Part model, mm, in its own coordinate system. Face numbers are marked on the shaded views. Coordinates: 2 decimals unless noted, no trailing zeros. Loops run counter-clockwise (first coordinate to the right, second up) from the corner with the lowest first, then second, coordinate; pieces in that order, holes last. Notation, with made-up numbers: (20.25, 4) -> (75.25, 4) arc R20 ccw to (75.25, 41) -> close; hole circle Ø10 at (23, -33.75). An arc over 180 degrees is marked (long way). One line per item, written item: value. Start each with the question number.
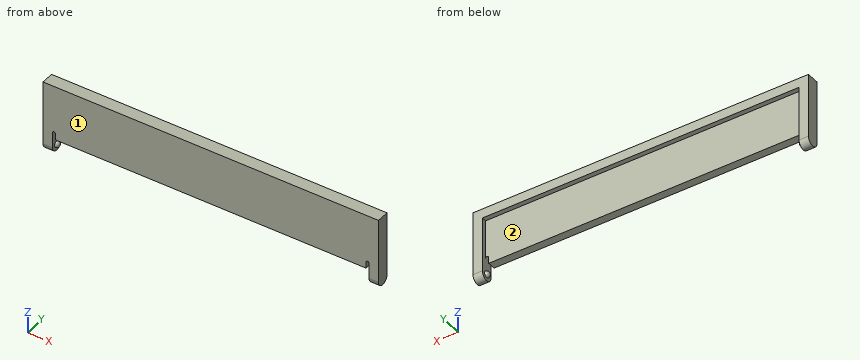
from build123d import *

# Parameters (mm, degrees)
SALIENTE_EXTRUIR1_DEPTH = 4
CROQUIS4_W              = 99
CROQUIS4_H              = 2
CORTAR_EXTRUIR1_DEPTH   = 10
REDONDEO1_R             = 2
CROQUIS5_W              = 101
CROQUIS5_H              = 16.071267716
CORTAR_EXTRUIR2_DEPTH   = 1.5


with BuildPart() as part:
    # Croquis1 → Saliente-Extruir1 (new body)
    with BuildSketch(Plane(origin=(0, 0, 0), x_dir=(1, 0, 0), z_dir=(0, 1, 0))):
        Polygon((-64.683943666, 30.054443615), (36.316056334, 30.054443615), (36.316056334, 33.054443615), (39.316056334, 33.054443615), (39.316056334, 30.054443615), (39.316056334, 10.554443615), (-67.683943666, 10.554443615), (-67.683943666, 30.054443615), (-67.683943666, 33.054443615), (-64.683943666, 33.054443615), align=None)
    extrude(amount=SALIENTE_EXTRUIR1_DEPTH)

    # Croquis4 → Cortar-Extruir1 (cut)
    with BuildSketch(Plane(origin=(0, 4, 0), x_dir=(1, 0, 0), z_dir=(0, 1, 0))):
        with Locations((-14.183943666, 29.054443615)):
            Rectangle(CROQUIS4_W, CROQUIS4_H)
        with BuildLine():
            Line((36.316056334, 26.054443615), (36.316056334, 30.054443615))
            Line((36.316056334, 30.054443615), (35.316056334, 30.054443615))
            Line((35.316056334, 30.054443615), (35.316056334, 28.054443615))
            Line((35.316056334, 28.054443615), (35.316056334, 26.054443615))
            ThreePointArc((35.316056334, 26.054443615), (35.816056334, 25.554443615), (36.316056334, 26.054443615))
        make_face()
        with BuildLine():
            Line((-63.683943666, 28.054443615), (-63.683943666, 30.054443615))
            Line((-63.683943666, 30.054443615), (-64.683943666, 30.054443615))
            Line((-64.683943666, 30.054443615), (-64.683943666, 26.054443615))
            ThreePointArc((-64.683943666, 26.054443615), (-64.183943666, 25.554443615), (-63.683943666, 26.054443615))
            Line((-63.683943666, 26.054443615), (-63.683943666, 28.054443615))
        make_face()
    extrude(amount=-CORTAR_EXTRUIR1_DEPTH, mode=Mode.SUBTRACT)

    # Redondeo1
    redondeo1_edges = [part.edges().sort_by_distance(p)[0] for p in [
        (-66.183943666, 0, -33.054443615),
        (-66.183943666, 4, -33.054443615),
        (37.816056334, 0, -33.054443615),
        (37.816056334, 4, -33.054443615),
    ]]
    fillet(redondeo1_edges, radius=REDONDEO1_R - 0.0001)  # a hair under: the kernel refuses the full size

    # Croquis3 → Revolución1 (revolve)
    with BuildSketch(Plane(origin=(-64.683943666, 0, 0), x_dir=(0, 0, -1), z_dir=(1, 0, 0))):
        with BuildLine():
            Line((32.054443615, 2), (30.054443615, 2))
            ThreePointArc((30.054443615, 2), (31.054443615, 1), (32.054443615, 2))
        make_face()
    revolve(axis=Axis((-64.683943666, 2, -32.054443615), (0, 0, 1)))

    # Croquis2 → Revolución2 (revolve)
    with BuildSketch(Plane.ZY.offset(-36.316056334)):
        with BuildLine():
            Line((-32.054443615, 2), (-30.054443615, 2))
            ThreePointArc((-30.054443615, 2), (-31.054443615, 1), (-32.054443615, 2))
        make_face()
    revolve(axis=Axis((36.316056334, 2, -32.054443615), (0, 0, 1)))

    # Croquis5 → Cortar-Extruir2 (cut)
    with BuildSketch(Plane(origin=(0, 4, 0), x_dir=(1, 0, 0), z_dir=(0, 1, 0))):
        with Locations((-14.183943666, 21.590077473)):
            Rectangle(CROQUIS5_W, CROQUIS5_H)
    extrude(amount=-CORTAR_EXTRUIR2_DEPTH, mode=Mode.SUBTRACT)


solid = part.part
1) Pin check, flat tips, straight feed: pin 1 Ø0.8 at (x, y) = (-31.5, 3.5) entering from -Z; pin 2 Ø2 at (x, z) = (15.5, -17) entering from -Y. Stop position of each tip, or through.
2) Pull direction X, two halves, no side cores. Call the marked faces 1 and 2: +X half, -X half, draft (parallel to the pull), parting line (faces both ways), or undercut.
3) Slice it at B-B (x = -31.5). Give the cut face in (y, z).
4) Probe line 1 (X direction, y = 2.65, z = -24); line 2 (Z direction, x = -7, y = 2.1); line 3 (Y direction, x = 22.5, z = -17). List the from-to ranges inside material, lowest first. Write a range as from..to.
5) Slice it at A-A (z = -27). Give the cut face in (x, y).
Check sheet entries:
1. pin 1: stops at z = -13.55
1. pin 2: stops at y = 0
2. face 1: draft
2. face 2: undercut
3. outline: (0, -28.05) -> (2.5, -28.05) -> (2.5, -13.55) -> (4, -13.55) -> (4, -10.55) -> (0, -10.55) -> close
4. line 1: x = -67.68..-64.68, 36.32..39.32
4. line 2: z = -28.05..-10.55
4. line 3: y = 0..2.5
5. outline: (-67.68, 0) -> (-64.68, 0) -> (-64.68, 4) -> (-67.68, 4) -> close; (-63.68, 0) -> (35.32, 0) -> (35.32, 2.5) -> (-63.68, 2.5) -> close; (36.32, 0) -> (39.32, 0) -> (39.32, 4) -> (36.32, 4) -> close
